from build123d import *

# Parameters (mm, degrees)
SKETCH2_R          = 1.5
CUT_EXTRUDE2_DEPTH = 7


with BuildPart() as part:
    # Sketch1 → Revolve1 (revolve)
    with BuildSketch(Plane.XY, mode=Mode.PRIVATE) as revolve1_sk:
        Polygon((0, 25.602357553), (0, 27.102357553), (-6.25, 27.102357553), (-6.25, 26.102357553), (-7, 26.102357553), (-7, 11.986662945), (-5.839130901, 11.986662945), (-5.11205907, 13.984276384), (-4.391648147, 15.963589129), (-4.391648147, 18.963589129), (-4.391648147, 22.963589129), align=None)
    revolve(revolve1_sk.sketch.rotate(Axis((0, -49.511916915, 0), (0, 1, 0)), 90), axis=Axis((0, -49.511916915, 0), (0, 1, 0)))

    # Sketch2 → Cut-Extrude2 (cut, symmetric)
    with BuildSketch(Plane.XY):
        with Locations((0, 18.986662945)):
            Circle(SKETCH2_R)
    extrude(amount=CUT_EXTRUDE2_DEPTH, both=True, mode=Mode.SUBTRACT)


solid = part.part
The model under review builds one solid part; all positions refer to its coordinate system, in mm. A direction names the side the tool comes from. Round coordinates to 2 decimals unless told otherwise and drop trailing zeros. Loops run counter-clockwise (first coordinate to the right, second up) from the corner with the lowest first, then second, coordinate; pieces in that order, holes last. Notation, with made-up numbers: (68, -35.75) -> (94, -35.75) arc R26 cw to (94, 3.25) -> close; hole circle Ø3 at (53, 14). An arc over 180 degrees is marked (long way). Write item = value, one per line. Start each with the question number.
Item 1: Take a section at D-D on y = 24. Give the boundary of the cut face in (x, z).
Item 2: Mouldability with a two-part tool opening along Y and no side actions: class faces 1 (the flat face through (0, 27.102, 0)), 2 (the cylindrical face through (-1.19, 18.074, 5.584)), 3 (the conical face through (-1, 25, 0)) as released by +Y, released by -Y, zero draft, split by the parting line, or undercut.
Item 3: To check wall thickness, follow L1, parallel to X at y = 17.5, z = 0; L2, parallel to Y at x = 0, z = 6.1; L3, parallel to Z at x = 1.25, y = 17.75. State the ranges of each line that lie inside material, in increasing order.
Item 4: Take a section at B-B on x = 1. Count the separate pieces of the cut face and the enclosed holes in it, plus the area to 3 significant figures.
Item 5: Take a section at A-A on y = 17.75. Give the boundary of the cut face in (x, z).
Item 6: Take a section at C-C on y = 22.25. Give the boundary of the cut face in (x, z), plus the area to 3 significant figures.
Item 7: For faces 4 (the cylindrical face through (-1.5, 19.05, -5.54)), 5 (the flat face through (6, 26.102, 3)), 6 (the cylindrical face through (-1.682, 19.513, 4.057)), list the 3-axis set-ups (+Z, -Z, +X, -X, +Y, -Y) from which the entire face can be reached by the end or side of a thin tool; tool diameter is ignored.
Item 8: Insertion check: pin 1 (5.5 mm diameter, centred on x = 0, z = 0, fed in from -Y); pin 2 (2 mm diameter, centred on y = 22.5, z = 4, fed in from +X); pin 3 (6 mm diameter, centred on y = 18.5, z = -5, fed in from -X). Each pin has a flat end and moves straight along its axis. Give the tip position at first contact, or say it passes through.
Result:
q1.outline = circle Ø14 at (0, 0); hole circle Ø5.33 at (0, 0)
q2.face_1 = released by +Y
q2.face_2 = undercut
q2.face_3 = released by -Y
q3.L1 = -7 to -4.39, 4.39 to 7
q3.L2 = 11.99 to 17.49, 20.49 to 27.1
q3.L3 = -6.89 to -4.21, 4.21 to 6.89
q4.separate_pieces = 3
q4.enclosed_holes = 0
q4.area = 86.3 mm²
q5.outline = (-0.85, -6.95) -> (-0.85, -4.31) arc R4.39 cw to (-0.85, 4.31) -> (-0.85, 6.95) arc R7 ccw to start; (0.85, -6.95) arc R7 ccw to (0.85, 6.95) -> (0.85, 4.31) arc R4.39 cw to (0.85, -4.31) -> close
q6.outline = circle Ø14 at (0, 0); hole circle Ø8.78 at (0, 0)
q6.area = 93.3 mm²
q7.face_4 = +Z, -Z
q7.face_5 = +Y
q7.face_6 = -Y
q8.pin_1 = 23.95
q8.pin_2 = 6.32
q8.pin_3 = -6.71
